Verification items for the finished model (mm, model axes). A direction names the side the tool comes from. Round coordinates to 2 decimals unless told otherwise and drop trailing zeros. Order: outer loops, then holes, each group sorted by start corner. A loop starts at its lowest first (then second) coordinate and runs counter-clockwise, first axis right, second up. Notation, with made-up numbers: (67.25, 74.5) -> (116.25, 74.5) arc R32 cw to (116.25, 105.5) -> close; hole circle Ø10 at (-12, 66.25). An arc over 180 degrees is marked (long way). Put each result on its own line as item: value.
```python
from build123d import *

# Parameters (mm, degrees)
F0_R     = 9.1
F0_R_2   = 3
F1_DEPTH = 3
F0_W     = 25
F0_H     = 4
F2_DEPTH = 32
F3_R     = 9.1
F3_R_2   = 3
F4_DEPTH = 3
F5_DEPTH = 1.2
F6_R     = 8.725
F7_DEPTH = 2
F8_DEPTH = 1.2


# Not quite as in the source:
# - a feature names something its author has since deleted; it is built from what else it names


with BuildPart() as f1:
    # F0 (on Front) → F1 (new body)
    with BuildSketch(Plane.XZ):
        with BuildLine():
            Line((55, 11.1), (-2.1, 11.1))
            ThreePointArc((-2.1, 11.1), (-8.4639610307, 8.4639610307), (-11.1, 2.1))
            Line((-11.1, 2.1), (-11.1, -2.1))
            ThreePointArc((-11.1, -2.1), (-8.4639610307, -8.4639610307), (-2.1, -11.1))
            Line((-2.1, -11.1), (30, -11.1))
            Line((30, -11.1), (30, -7.1))
            Line((30, -7.1), (55, -7.1))
            Line((55, -7.1), (55, 11.1))
        make_face()
        Circle(F0_R, mode=Mode.SUBTRACT)
        Circle(F0_R)
        Circle(F0_R_2, mode=Mode.SUBTRACT)
    extrude(amount=-F1_DEPTH)

    # F0 (on Front) → F2 (join)
    with BuildSketch(Plane.XZ):
        Polygon((59, 11.1), (55, 11.1), (55, -7.1), (55, -11.1), (59, -11.1), align=None)
        with Locations((42.5, -9.1)):
            Rectangle(F0_W, F0_H)
    extrude(amount=-F2_DEPTH)

    # F3 (on face) → F4 (join)
    with BuildSketch(Plane(origin=(0, 32, 0), x_dir=(-1, 0, 0), z_dir=(0, 1, 0))):
        with BuildLine():
            Line((-30, -7.1), (-30, -11.1))
            Line((-30, -11.1), (2.1, -11.1))
            ThreePointArc((2.1, -11.1), (8.4639610307, -8.4639610307), (11.1, -2.1))
            Line((11.1, -2.1), (11.1, 2.1))
            ThreePointArc((11.1, 2.1), (8.4639610307, 8.4639610307), (2.1, 11.1))
            Line((2.1, 11.1), (-55, 11.1))
            Line((-55, 11.1), (-55, -7.1))
            Line((-55, -7.1), (-30, -7.1))
        make_face()
        Circle(F3_R, mode=Mode.SUBTRACT)
        Circle(F3_R)
        Circle(F3_R_2, mode=Mode.SUBTRACT)
    extrude(amount=-F4_DEPTH)

    # F0 (on Front) → F5 (cut)
    with BuildSketch(Plane.XZ):
        Circle(F0_R)
        Circle(F0_R_2, mode=Mode.SUBTRACT)
    extrude(amount=-F5_DEPTH, mode=Mode.SUBTRACT)

    # F6 (on face) → F7 (cut)
    with BuildSketch(Plane.YZ.offset(59)):
        with Locations((16, 0)):
            Circle(F6_R)
    extrude(amount=-F7_DEPTH, mode=Mode.SUBTRACT)

    # F3 (on face) → F8 (cut)
    with BuildSketch(Plane(origin=(0, 32, 0), x_dir=(-1, 0, 0), z_dir=(0, 1, 0))):
        Circle(F3_R)
        Circle(F3_R_2, mode=Mode.SUBTRACT)
    extrude(amount=-F8_DEPTH, mode=Mode.SUBTRACT)


solid = f1.part
```
Item 1: Tool access check on faces 5 (the face through (0, 1.2, -4)), 6 (the face through (57, 16, 0)), 7 (the face through (37, 30, 11.1)), 8 (the face through (21, 3, 0)). Record the directions out of +Z, -Z, +X, -X, +Y, -Y that give a thin tool (end or side, any length) a straight path to the whole face; none if there is none.
Geometry check:
face 5: -Y
face 6: +X
face 7: +Z, +X, -X, +Y, -Y
face 8: +Z, -X
Item 2: Sectioned sample at D-D, the plane y = 16. Record the boundary of the cut face in (x, z) (3 decimals), then the cut area to 3 significant figures.
Geometry check:
outline: (30, -11.1) -> (59, -11.1) -> (59, -8.725) -> (57, -8.725) -> (57, 8.725) -> (59, 8.725) -> (59, 11.1) -> (55, 11.1) -> (55, -7.1) -> (30, -7.1) -> close
area: 154 mm2
Item 3: Sectioned sample at B-B, the plane x = 12. Record the boundary of the cut face in (y, z).
Geometry check:
outline: (0, -11.1) -> (3, -11.1) -> (3, 11.1) -> (0, 11.1) -> close; (29, -11.1) -> (32, -11.1) -> (32, 11.1) -> (29, 11.1) -> close
Item 4: Sectioned sample at A-A, the plane x = 0. Record the boundary of the cut face in (y, z).
Geometry check:
outline: (0, -11.1) -> (3, -11.1) -> (3, -3) -> (1.2, -3) -> (1.2, -9.1) -> (0, -9.1) -> close; (0, 9.1) -> (1.2, 9.1) -> (1.2, 3) -> (3, 3) -> (3, 11.1) -> (0, 11.1) -> close; (29, -11.1) -> (32, -11.1) -> (32, -9.1) -> (30.8, -9.1) -> (30.8, -3) -> (29, -3) -> close; (29, 3) -> (30.8, 3) -> (30.8, 9.1) -> (32, 9.1) -> (32, 11.1) -> (29, 11.1) -> close
Item 5: Depth check by flat-ended pin: pin 1 Ø12 at (y, z) = (22, -5) entering from +X; pin 2 Ø5 at (x, z) = (0, 0) entering from +Y; pin 3 Ø12 at (y, z) = (17, -5.5) entering from -X; pin 4 Ø1.5 at (y, z) = (7.5, 1.5) entering from -X. Enter the tip coordinate at first touch or a pass-through.
Geometry check:
pin 1: x = 59
pin 2: through
pin 3: x = 30
pin 4: x = 55
Item 6: Sectioned sample at C-C, the plane z = 0. Record the boundary of the cut face in (x, y) (3 decimals), then the cut area to 3 significant figures.
Geometry check:
outline: (-11.1, 0) -> (-9.1, 0) -> (-9.1, 1.2) -> (-3, 1.2) -> (-3, 3) -> (-11.1, 3) -> close; (-11.1, 29) -> (-3, 29) -> (-3, 30.8) -> (-9.1, 30.8) -> (-9.1, 32) -> (-11.1, 32) -> close; (3, 1.2) -> (9.1, 1.2) -> (9.1, 0) -> (59, 0) -> (59, 7.275) -> (57, 7.275) -> (57, 24.725) -> (59, 24.725) -> (59, 32) -> (9.1, 32) -> (9.1, 30.8) -> (3, 30.8) -> (3, 29) -> (55, 29) -> (55, 3) -> (3, 3) -> close
area: 424 mm2
Item 7: Material ranges on line 1 along Y through (x, z) = (52, 5.75); line 2 along Z through (x, y) = (0, 1); line 3 along Z through (x, y) = (0, 30), recorded low to high.
Geometry check:
line 1: 0 to 3, 29 to 32
line 2: -11.1 to -9.1, 9.1 to 11.1
line 3: -11.1 to -3, 3 to 11.1
Item 8: Release check for a two-part mould opening along X. For faces 1 (the face through (31, 0, 0)), 2 (the face through (-8.394, 30.521, -8.534)), 3 (the face through (0, 30.8, -4)), 4 (the face through (1.973, 31.408, -8.884)) record: pulls with the +X half, pulls with the -X half, needs draft (parallel to the pull), parting line crosses it, or undercut.
Geometry check:
face 1: needs draft
face 2: pulls with the -X half
face 3: undercut
face 4: undercut
